```python
from build123d import *

# Parameters (mm, degrees)
SKETCH_1_W          = 8
SKETCH_1_H          = 8
EXTRUDE_1_DEPTH     = 34
SKETCH_2_R          = 1.6
CUT_EXTRUDE_1_DEPTH = 35
SKETCH_3_R          = 1.6
CUT_EXTRUDE_2_DEPTH = 34
SKETCH_4_R          = 1.6
CUT_EXTRUDE_3_DEPTH = 34


with BuildPart() as part:
    # 草图1 → 凸台-拉伸1 (new body)
    with BuildSketch(Plane.XY):
        with Locations((5.832511347, 6.305290853)):
            Rectangle(SKETCH_1_W, SKETCH_1_H)
    extrude(amount=EXTRUDE_1_DEPTH)

    # 草图2 → 切除-拉伸1 (cut, through all)
    with BuildSketch(Plane.XY.offset(34)):
        with Locations((5.832511347, 6.305290853)):
            Circle(SKETCH_2_R)
    extrude(amount=-CUT_EXTRUDE_1_DEPTH, mode=Mode.SUBTRACT)

    # 草图3 → 切除-拉伸2 (cut)
    with BuildSketch(Plane(origin=(0, 10.305290853, 0), x_dir=(1, 0, 0), z_dir=(0, 1, 0))):
        with Locations((5.832511347, -13)):
            Circle(SKETCH_3_R)
        with Locations((5.832511347, -21)):
            Circle(SKETCH_3_R)
    extrude(amount=-CUT_EXTRUDE_2_DEPTH, mode=Mode.SUBTRACT)

    # 草图4 → 切除-拉伸3 (cut)
    with BuildSketch(Plane(origin=(9.832511347, 0, 0), x_dir=(0, 0, -1), z_dir=(1, 0, 0))):
        with Locations((-26, 6.305290853)):
            Circle(SKETCH_4_R)
        with Locations((-8, 6.305290853)):
            Circle(SKETCH_4_R)
    extrude(amount=-CUT_EXTRUDE_3_DEPTH, mode=Mode.SUBTRACT)


solid = part.part
```
The listing builds one solid part. Answer for the finished solid, in the listing's coordinates (mm). Coordinates: 2 decimals unless noted, no trailing zeros. Write each loop counter-clockwise with the first axis right and the second up, starting at its lowest first coordinate (ties: lowest second). Pieces come first, ordered by that corner, then holes. Notation, with made-up numbers: (49.25, -13) - (73.25, -13) arc R23 cw to (73.25, 23) - close; hole circle Ø5 at (65, 12). An arc over 180 degrees is marked (long way). One line per item, written item: value.
1) This flat-tipped pin is pushed along its axis until it touches: pin 1 Ø1.9 at (x, z) = (5.83, 21) entering from -Y. Where does it stop, or does it pass through?
Geometry check:
pin 1: passes through
2) Find section D-D (y = 7). Count the separate pieces of the cut face and the enclosed holes in it, and give its area (3 significant figures).
Geometry check:
separate pieces: 6
enclosed holes: 0
area: 144 mm2
3) Find section C-C (z = 25.5). Give the vertices of the cut face in (x, y).
Geometry check:
outline: (1.83, 2.31) - (9.83, 2.31) - (9.83, 4.79) - (6.33, 4.79) arc R1.6 cw to (5.33, 4.79) - (1.83, 4.79) - close; (1.83, 7.83) - (5.33, 7.83) arc R1.6 cw to (6.33, 7.83) - (9.83, 7.83) - (9.83, 10.31) - (1.83, 10.31) - close
4) Find section A-A (z = 31). Give the vertices of the cut face in (x, y), and give its area (3 significant figures).
Geometry check:
outline: (1.83, 2.31) - (9.83, 2.31) - (9.83, 10.31) - (1.83, 10.31) - close; hole circle Ø3.2 at (5.83, 6.31)
area: 56.0 mm2
5) Find section B-B (x = 3.75). Give the vertices of the cut face in (y, z), and give its area (3 significant figures).
Geometry check:
outline: (2.31, 0) - (10.31, 0) - (10.31, 34) - (2.31, 34) - close; hole circle Ø3.2 at (6.31, 8); hole circle Ø3.2 at (6.31, 26)
area: 256 mm2
6) Consider line 1 along X through (y, z) = (4.9, 21); line 2 along Z through (x, y) = (7.25, 9.75); line 3 along Z through (x, y) = (3.25, 7.5). Determine where each line is inside the solid, lowest interval first. Write a range as from..to.
Geometry check:
line 1: x = 1.83..4.23, 7.43..9.83
line 2: z = 0..12.26, 13.74..20.26, 21.74..34
line 3: z = 0..6.94, 9.06..24.94, 27.06..34
7) For a pull along Y with two mould halves and no side action, classify faces 1 (the flat face through (6, 2.305, 17)), 2 (the flat face through (1.833, 6, 17)), 3 (the cylindrical face through (5.62, 7.89, 10.54)) as pulls with the +Y half, pulls with the -Y half, needs draft (parallel to the pull), parting line crosses it, or undercut.
Geometry check:
face 1: pulls with the -Y half
face 2: needs draft
face 3: undercut
